from build123d import *

# Parameters (mm, degrees)
SKETCH_1_R      = 1.5
SKETCH_1_W      = 8.2
SKETCH_1_H      = 2.2
SKETCH_1_W_2    = 94
SKETCH_1_H_2    = 50.875
EXTRUDE_1_DEPTH = 2


with BuildPart() as part:
    # 草图1 → 凸台-拉伸1 (new body)
    with BuildSketch(Plane.XY):
        Polygon((-62.766155614, -54.699512395), (-62.766155614, -53.199512395), (-65.266155614, -53.199512395), (-65.266155614, -79.137012395), (-67.266155614, -79.137012395), (-67.266155614, -87.137012395), (-65.266155614, -87.137012395), (-65.266155614, -118.574512395), (60.733844386, -118.574512395), (60.733844386, -87.137012395), (62.733844386, -87.137012395), (62.733844386, -79.137012395), (60.733844386, -79.137012395), (60.733844386, -53.199512395), (58.233844386, -53.199512395), (58.233844386, -54.699512395), (55.633844386, -54.699512395), (55.633844386, -53.199512395), (52.633844386, -53.199512395), (52.633844386, -50.199512395), (55.633844386, -50.199512395), (55.633844386, -48.699512395), (58.233844386, -48.699512395), (58.233844386, -50.199512395), (60.733844386, -50.199512395), (60.733844386, -31.699512395), (-65.266155614, -31.699512395), (-65.266155614, -50.199512395), (-62.766155614, -50.199512395), (-62.766155614, -48.699512395), (-60.166155614, -48.699512395), (-60.166155614, -50.199512395), (-57.166155614, -50.199512395), (-57.166155614, -53.199512395), (-60.166155614, -53.199512395), (-60.166155614, -54.699512395), align=None)
        with Locations((-35.266155614, -114.574512396)):
            Circle(SKETCH_1_R, mode=Mode.SUBTRACT)
        with Locations((-20.016155614, -114.574512396)):
            Rectangle(SKETCH_1_W, SKETCH_1_H, mode=Mode.SUBTRACT)
        with Locations((15.483844386, -114.574512396)):
            Rectangle(SKETCH_1_W, SKETCH_1_H, mode=Mode.SUBTRACT)
        with Locations((30.733844386, -114.574512396)):
            Circle(SKETCH_1_R, mode=Mode.SUBTRACT)
        with Locations((-2.266155614, -75.137012395)):
            Rectangle(SKETCH_1_W_2, SKETCH_1_H_2, mode=Mode.SUBTRACT)
    extrude(amount=EXTRUDE_1_DEPTH)


solid = part.part
The model under review builds one solid part; all positions refer to its coordinate system, in mm. Give positions to 0.01 mm unless a question says otherwise; leave off trailing zeros. Order: outer loops, then holes, each group sorted by start corner. A loop starts at its lowest first (then second) coordinate and runs counter-clockwise, first axis right, second up. Notation, with made-up numbers: M -11,35 L 17,35 A22 cw 17,43 Z; hole C -26.5,53.5 d5. An arc over 180 degrees is marked long. One line per question, with ' | ' between items. Start each with the question number.
1) Consider section B-B, the plane y = -91.5. Give the boundary of the cut face in (x, z).
2) Clearance check with flat-ended pins moving along their axes: P1, Ø1, axis at y = -67.5, z = 1.5, coming from the -X side; P2, Ø0.6, axis at y = -114.5, z = 1, coming from the +X side; P3, Ø1, axis at x = 61.5, z = 0.5, coming from the +Y side; P4, Ø12, axis at x = -43, y = -74.5, coming from the -Z side. State where each tip first meets the part, or that it passes through.
3) Wall thickness on L1, parallel to X at y = -50, z = 0.3; L2, parallel to Y at x = -29.5, z = 1.15; L3, parallel to X at y = -72, z = 1.85: over which ranges is each line inside the solid? List them lowest first. Write a range as from..to.
4) Consider section A-A, the plane x = -7. Give the boundary of the cut face in (y, z), then the cut area to 3 significant figures.
5) Consider section C-C, the plane z = 1.5. State how many separate pieces and enclosed holes the cut face has, then the cut area to 3 significant figures.
6) Mouldability with a two-part tool opening along Y and no side actions: class faces 1 (the face through (-34.574, -115.905, 0.986)), 2 (the face through (-3, -103, 2)), 3 (the face through (31.426, -115.905, 0.986)) as pulls with the +Y half, pulls with the -Y half, needs draft (parallel to the pull), parting line crosses it, or undercut.
Found:
1) outline: M -65.27,0 L -49.27,0 L -49.27,2 L -65.27,2 Z; M 44.73,0 L 60.73,0 L 60.73,2 L 44.73,2 Z
2) P1: stops at x = -65.27 | P2: stops at x = 60.73 | P3: stops at y = -79.14 | P4: passes through
3) L1: x = -65.27..-62.77, -60.17..-49.27, 44.73..55.63, 58.23..60.73 | L2: y = -118.57..-100.57, -49.7..-31.7 | L3: x = -65.27..-49.27, 44.73..60.73
4) outline: M -118.57,0 L -100.57,0 L -100.57,2 L -118.57,2 Z; M -49.7,0 L -31.7,0 L -31.7,2 L -49.7,2 Z | area: 72.0 mm²
5) separate pieces: 1 | enclosed holes: 5 | area: 6,080 mm²
6) face 1: undercut | face 2: needs draft | face 3: undercut
